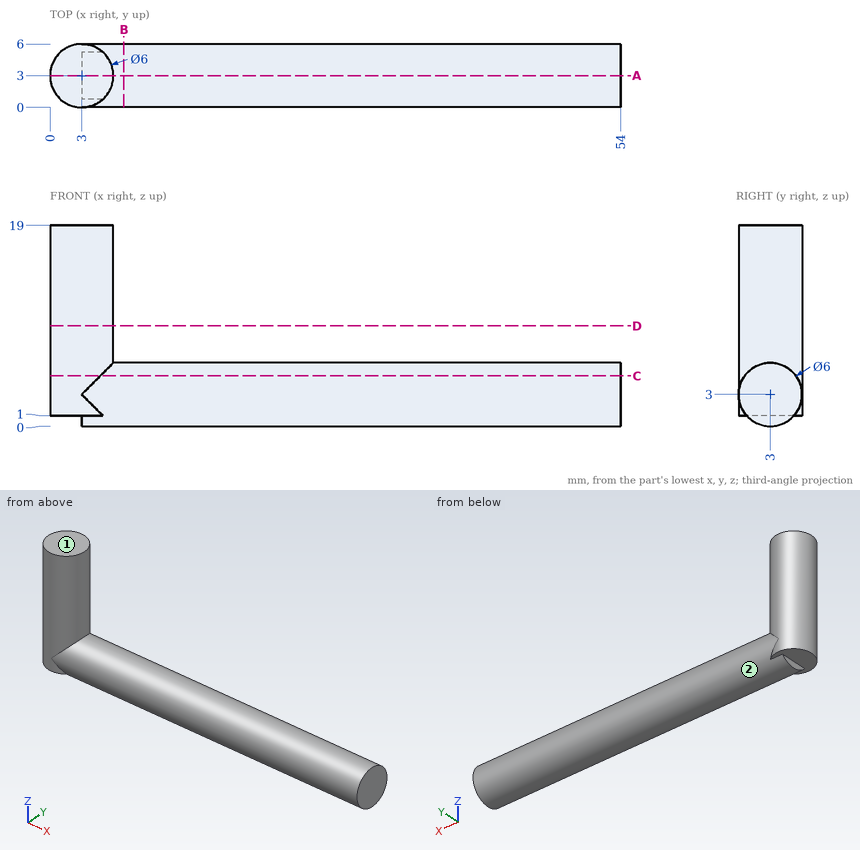
Verification items for this drawing (mm, ordinates from the low corner). A direction names the side the tool comes from. Give positions to 0.01 mm unless a question says otherwise; leave off trailing zeros. Loops run counter-clockwise (first coordinate to the right, second up) from the corner with the lowest first, then second, coordinate; pieces in that order, holes last.
1. Material ranges on probe 1 along Z at (x, y) = (51, 3.15); probe 2 along X at (y, z) = (3.1, 5); probe 3 along X at (y, z) = (3.3, 17), recorded low to high.
Derived:
probe 1: z = 0 to 6
probe 2: x = 0 to 54
probe 3: x = 0.02 to 5.98
2. Cross-section at B-B on x = 7. Record the cut outline in (y, z), and give its area (3 significant figures).
Derived:
outline: circle Ø6 at (3, 3)
area: 28.3 mm2
3. Cross-section at A-A on y = 3. Record the cut outline in (x, z), and give its area (3 significant figures).
Derived:
outline: (0, 1) - (3, 1) - (3, 0) - (54, 0) - (54, 6) - (6, 6) - (6, 19) - (0, 19) - close
area: 399 mm2
4. Cross-section at C-C on z = 4.75. Record the cut outline in (x, y).
Derived:
outline: (4.75, 0.56) - (54, 0.56) - (54, 5.44) - (4.75, 5.44) arc R3 ccw (long way) to start
5. Go/stop test with flat-tipped pins: P1, Ø1, axis at y = 2, z = 11, coming from the -X side; P2, Ø0.8, axis at y = 3, z = 0.5, coming from the -X side; P3, Ø1.5, axis at y = 4.5, z = 16.5, coming from the -X side; P4, Ø1.5, axis at x = 21.5, z = 8.5, coming from the -Y side. Record where each tip stops, or that it passes through.
Derived:
P1: stops at x = 0.04
P2: stops at x = 3
P3: stops at x = 0.1
P4: passes through
6. Tool access check on the marked faces 1 and 2. Record the directions out of +Z, -Z, +X, -X, +Y, -Y that give a thin tool (end or side, any length) a straight path to the whole face; none if there is none.
Derived:
face 1: +Z, +X, -X, +Y, -Y
face 2: +X
